For this review, take the finished solid that the model builds, in its own axes (mm). A direction names the side the tool comes from. Coordinates: 2 decimals unless noted, no trailing zeros. Answer in a Markdown table with one row per item.
from build123d import *

# Parameters (mm, degrees)
BODY_DEPTH  = 20
BODY_TAPER  = 8
SKETCH2_R   = 1.5
SCREW_DEPTH = 8


with BuildPart() as part:
    # Sketch1 → Body (new body)
    with BuildSketch(Plane(origin=(0, 0, 0), x_dir=(1, 0, 0), z_dir=(0, 1, 0))):
        with BuildLine():
            ThreePointArc((2.5, -12.5), (9.571067812, -9.571067812), (12.5, -2.5))
            Line((12.5, -2.5), (12.5, 2.5))
            ThreePointArc((12.5, 2.5), (9.571067812, 9.571067812), (2.5, 12.5))
            Line((2.5, 12.5), (-2.5, 12.5))
            ThreePointArc((-2.5, 12.5), (-9.571067812, 9.571067812), (-12.5, 2.5))
            Line((-12.5, 2.5), (-12.5, -2.5))
            ThreePointArc((-12.5, -2.5), (-9.571067812, -9.571067812), (-2.5, -12.5))
            Line((-2.5, -12.5), (2.5, -12.5))
        make_face()
    extrude(amount=BODY_DEPTH, taper=BODY_TAPER)

    # Sketch2 → Screw (cut)
    with BuildSketch(Plane(origin=(0, 20, 0), x_dir=(1, 0, 0), z_dir=(0, 1, 0))):
        with Locations(Location((0, 0, 0), (0, 0, 270))):
            Circle(SKETCH2_R)
    extrude(amount=-SCREW_DEPTH, mode=Mode.SUBTRACT)


solid = part.part
Item 1: For L1, parallel to X at y = 18.75, z = 0; L2, parallel to Z at x = -0.75, y = 17.25; L3, parallel to X at y = 15, z = 0, list the stretches that pass through material, from the lowest coordinate up.
Worked answers:
| item | result |
|---|---|
| L1 | -9.86 to -1.5, 1.5 to 9.86 |
| L2 | -10.08 to -1.3, 1.3 to 10.08 |
| L3 | -10.39 to -1.5, 1.5 to 10.39 |
Item 2: The part is to be moulded in two halves that separate along X. For faces 1 (the conical face through (8.63, 10.14, -8.496)), 2 (the conical face through (-8.63, 10.14, 8.496)), 3 (the cylindrical face through (0.45, 16.06, 1.43)), say which applies: +X half, -X half, draft (parallel to the pull), parting line (faces both ways), or undercut.
Worked answers:
| item | result |
|---|---|
| face 1 | +X half |
| face 2 | -X half |
| face 3 | undercut |
Item 3: Insertion check: pin 1 (12 mm diameter, centred on y = 12.5, z = -9, fed in from -X); pin 2 (6 mm diameter, centred on x = 4, y = 8.5, fed in from -Z); pin 3 (0.9 mm diameter, centred on x = -0.5, z = -0.5, fed in from +Y). Each pin has a flat end and moves straight along its axis. Give the tip position at first contact, or say it passes through.
Worked answers:
| item | result |
|---|---|
| pin 1 | x = -11.08 |
| pin 2 | z = -11.69 |
| pin 3 | y = 12 |
Item 4: For faces 4 (the flat face through (0, 0, 0)), 5 (the flat face through (0, 12, 0)), list the 3-axis set-ups (+Z, -Z, +X, -X, +Y, -Y) from which the entire face can be reached by the end or side of a thin tool; tool diameter is ignored.
Worked answers:
| item | result |
|---|---|
| face 4 | +Z, -Z, +X, -X, -Y |
| face 5 | +Y |
